```python
from build123d import *

# Parameters (mm, degrees)
SKETCH1_R           = 5.75
BOSS_EXTRUDE1_DEPTH = 25
SKETCH2_R           = 3.341548393
CUT_EXTRUDE1_DEPTH  = 15
CUT_EXTRUDE2_DEPTH  = 8
CIRPATTERN1_COUNT   = 3
CUT_EXTRUDE3_DEPTH  = 8
SKETCH7_R           = 0.9
CUT_EXTRUDE4_DEPTH  = 0.1


with BuildPart() as part:
    # Sketch1 → Boss-Extrude1 (new body)
    with BuildSketch(Plane(origin=(0, 0, 0), x_dir=(1, 0, 0), z_dir=(0, 1, 0))):
        with Locations(Location((0, 0, 0), (0, 0, 270))):
            Circle(SKETCH1_R)
    extrude(amount=BOSS_EXTRUDE1_DEPTH)

    # Sketch2 → Cut-Extrude1 (cut)
    with BuildSketch(Plane(origin=(0, 0, 0), x_dir=(1, 0, 0), z_dir=(0, 1, 0))):
        with Locations(Location((0, 0, 0), (0, 0, 270))):
            Circle(SKETCH2_R)
    extrude(amount=CUT_EXTRUDE1_DEPTH, mode=Mode.SUBTRACT)

    # Sketch5 → Cut-Extrude2 (cut)
    with BuildSketch(Plane(origin=(0, 0, 0), x_dir=(1, 0, 0), z_dir=(0, 1, 0))):
        with BuildLine():
            Line((-1.035655919, -3.177005269), (-1.933412335, -5.415202373))
            ThreePointArc((-1.933412335, -5.415202373), (0, -5.75), (1.933412335, -5.415202373))
            Line((1.933412335, -5.415202373), (1.035655919, -3.177005269))
            ThreePointArc((1.035655919, -3.177005269), (0, -3.341548393), (-1.035655919, -3.177005269))
        make_face()
    cut_extrude2 = extrude(amount=CUT_EXTRUDE2_DEPTH, mode=Mode.SUBTRACT)

    # CirPattern1: Cut-Extrude2 ×3 about axis
    cirpattern1_axis = Axis((0, 0, 0), (0, 1, 0))
    for i in range(1, CIRPATTERN1_COUNT):
        add(cut_extrude2.rotate(cirpattern1_axis, i * 360 / CIRPATTERN1_COUNT), mode=Mode.SUBTRACT)

    # Sketch6 → Cut-Extrude3 (cut)
    with BuildSketch(Plane(origin=(0, 25, 0), x_dir=(1, 0, 0), z_dir=(0, 1, 0))):
        with BuildLine():
            Line((0.41, 2.964671599), (0.41, -2.964671599))
            ThreePointArc((0.41, -2.964671599), (3.374671599, 0), (0.41, 2.964671599))
        make_face()
        with BuildLine():
            Line((-0.416408681, 2.965564682), (-0.416408681, -2.965564682))
            ThreePointArc((-0.416408681, -2.965564682), (-3.381973363, 0), (-0.416408681, 2.965564682))
        make_face()
    extrude(amount=-CUT_EXTRUDE3_DEPTH, mode=Mode.SUBTRACT)

    # Sketch7 → Cut-Extrude4 (cut)
    with BuildSketch(Plane.XZ.offset(-15)):
        with Locations(Location((0, 0, 0), (0, 0, 270))):
            Circle(SKETCH7_R)
    extrude(amount=-CUT_EXTRUDE4_DEPTH, mode=Mode.SUBTRACT)


solid = part.part
```
CAD build for the part. Positions are in the model's coordinates, mm. A direction names the side the tool comes from. Round coordinates to 2 decimals unless told otherwise and drop trailing zeros. Order: outer loops, then holes, each group sorted by start corner. A loop starts at its lowest first (then second) coordinate and runs counter-clockwise, first axis right, second up.
Item 1: Saw through at A-A on y = 3. Write the cut outline in (x, z), then the cut area to 3 significant figures.
Item 2: Pin check, flat tips, straight feed: pin 1 (1.4 mm diameter, centred on x = 0, z = 0, fed in from -Y); pin 2 (1 mm diameter, centred on x = -4.5, z = -3, fed in from -Y); pin 3 (0.9 mm diameter, centred on x = -0.5, z = 0, fed in from -Y). Stop position of each tip, or through.
Item 3: Saw through at D-D on y = 14.5. Write the cut outline in (x, z), then the cut area to 3 significant figures.
Item 4: Saw through at C-C on x = 0. Write the cut outline in (y, z).
Item 5: Mould opens along Z. For faces 1 (the face through (0, 0, -4)), 2 (the face through (-1.48, 3.94, 4.28)), 3 (the face through (-0.416, 21, 0)) say: pulls with the +Z half, pulls with the -Z half, needs draft (parallel to the pull), parting line crosses it, or undercut.
Item 6: Probe line 1 along X through (y, z) = (18.25, 0.5); line 2 along Z through (x, y) = (0, 10.5); line 3 along Z through (x, y) = (1.25, 2.25). List the from-to ranges inside material, lowest first.
Item 7: Saw through at B-B on z = 0. Write the cut outline in (x, y), then the cut area to 3 significant figures.
Item 8: Tool access for faces 4 (the face through (3.374, 21.056, 0.065)), 5 (the face through (0, 8, 5)), 6 (the face through (-2.97, 3.94, -3.42)): list every direction of +Z, -Z, +X, -X, +Y, -Y with a clear straight run to the whole face (end or side of a thin tool).
Reported:
1. outline: (-5.66, -1.03) - (-3.27, -0.69) arc R3.34 cw to (-1.04, 3.18) - (-1.93, 5.42) arc R5.75 ccw to start; (-3.72, -4.38) arc R5.75 ccw to (3.72, -4.38) - (2.23, -2.49) arc R3.34 cw to (-2.23, -2.49) - close; (1.04, 3.18) arc R3.34 cw to (3.27, -0.69) - (5.66, -1.03) arc R5.75 ccw to (1.93, 5.42) - close
1. area: 46.9 mm2
2. pin 1: stops at y = 15.1
2. pin 2: stops at y = 8
2. pin 3: stops at y = 15
3. outline: circle Ø11.5 at (0, 0); hole circle Ø6.68 at (0, 0)
3. area: 68.8 mm2
4. outline: (0, -5.75) - (25, -5.75) - (25, 5.75) - (8, 5.75) - (8, 3.34) - (15, 3.34) - (15, 0.9) - (15.1, 0.9) - (15.1, -0.9) - (15, -0.9) - (15, -3.34) - (0, -3.34) - close
5. face 1: needs draft
5. face 2: pulls with the +Z half
5. face 3: undercut
6. line 1: x = -5.73 to -3.34, -0.42 to 0.41, 3.33 to 5.73
6. line 2: z = -5.75 to -3.34, 3.34 to 5.75
6. line 3: z = -5.61 to -3.1, 3.1 to 3.71
7. outline: (-5.75, 0) - (-3.34, 0) - (-3.34, 15) - (-0.9, 15) - (-0.9, 15.1) - (0.9, 15.1) - (0.9, 15) - (3.34, 15) - (3.34, 0) - (5.75, 0) - (5.75, 25) - (3.37, 25) - (3.37, 17) - (0.41, 17) - (0.41, 25) - (-0.42, 25) - (-0.42, 17) - (-3.38, 17) - (-3.38, 25) - (-5.75, 25) - close
7. area: 140 mm2
8. face 4: +Y
8. face 5: +Z, -Y
8. face 6: -X, -Y
